Can you work these out from the model? Positions are in its coordinate system, mm. A direction names the side the tool comes from. Coordinates: 2 decimals unless noted, no trailing zeros. Order: outer loops, then holes, each group sorted by start corner. A loop starts at its lowest first (then second) coordinate and runs counter-clockwise, first axis right, second up. Notation, with made-up numbers: M -35.5,13 L -21.5,13 A10 cw -21.5,27 Z; hole C -27.5,81 d3. An arc over 180 degrees is marked long. Answer as CSV lines item,"result". Start each with the question number.
1. If we section it at A-A (x = -3.25): List the corners of the cut face in (y, z) for me, plus the area to 3 significant figures.
2. Will these pins go through, and if not, where does the flat tip stop? pin 1 (1 mm diameter, centred on x = 4.5, z = -0.5, fed in from -Y); pin 2 (0.5 mm diameter, centred on y = 1, z = -1.5, fed in from -X); pin 3 (1 mm diameter, centred on y = 3, z = 1, fed in from +X).
3. If we section it at B-B (x = 2.25): List the corners of the cut face in (y, z) for me, plus the area to 3 significant figures.
4. If we mould it in two halves opening along Z, with no side actions, what happens to faces 4 (the face through (-3.77, 1.74, 0.99)), 5 (the face through (-2.218, 2.285, 3.584)), 6 (the face through (-5, -2, 1))? For each: released by +Z, released by -Z, zero draft, split by the parting line, or undercut.
5. On a 3-axis mill with a long thin cutter (end or side, diameter ignored), from which of +Z, -Z, +X, -X, +Y, -Y can I reach the whole of each face in a straight line? I mean faces 1 (the face through (0, 0, -3)), 2 (the face through (-4, 0, 2)), 3 (the face through (8, 0, 0)). Say none if no direction works.
6. I need wall thicknesses on line 1 along Y through (x, z) = (-3.25, -1.75); line 2 along Z through (x, y) = (-2.75, -1); line 3 along X through (y, z) = (-2.25, 1.5). Which ranges of each line are inside material? Lowest first, please. Write a range as from..to.
Autodesk Inventor part; units mm, degrees
ref_plane "bolt_XY" through (0, 0, 0) normal (1, 0, 0) x (0, 0, -1)
ref_plane "bolt_YZ" through (0, 0, 0) normal (0, 0, -1) x (0, 1, 0)
ref_plane "bolt_ZX" through (0, 0, 0) normal (0, 1, 0) x (1, 0, 0)
sketch "Sketch_8" plane through (0, 0, 0) normal (0, 0, 1) x (1, 0, 0)
  line L0 (8, 0) -> (-5, 0)
  line L1 (-5, 0) -> (-5, 3.9613)
  line L2 (-5, 3.9613) -> (-4.5, 4.25)
  line L3 (-4.5, 4.25) -> (0, 4.25)
  line L4 (0, 4.25) -> (0, 2.7)
  arc A0 (0, 2.7) -> (0.2, 2.5) centre (0.2, 2.7) ccw
  line L5 (0.2, 2.5) -> (7.5095, 2.5)
  line L6 (7.5095, 2.5) -> (8, 2.0095)
  line L7 (8, 2.0095) -> (8, 0)
  line L8 (8, 0) -> (-5, 0)
revolve "Revolution1" add sketch "Sketch_8" angle 360 about axis through (8, 0, 0) along (1, 0, 0)
thread "Thread1"
sketch "Sketch2" plane through (-5, 0, 0) normal (-1, 0, 0) x (0, 0, 1)
  point P0 (0, 0)
hole "Hole1" at (-5, 0, 0) direction (1, 0, 0) diameter 4 depth 2.5 tip angle 120
sketch "Sketch_3" plane through (-5, 0, 0) normal (1, 0, 0) x (0, 0, -1)
  line L0 (-2, -1.1547) -> (0, -2.3094)
  line L1 (0, -2.3094) -> (2, -1.1547)
  line L2 (2, -1.1547) -> (2, 1.1547)
  line L3 (2, 1.1547) -> (0, 2.3094)
  line L4 (0, 2.3094) -> (-2, 1.1547)
  line L5 (-2, 1.1547) -> (-2, -1.1547)
extrude "Extrusion1" cut sketch "Sketch_3" along normal blind 2.5
ref_plane "bolt_XY" through (0, 0, 0) normal (1, 0, 0) x (0, 0, -1)
ref_plane "bolt_YZ" through (0, 0, 0) normal (0, 0, -1) x (0, 1, 0)
ref_plane "bolt_ZX" through (0, 0, 0) normal (0, 1, 0) x (1, 0, 0)
ref_plane "nut_XY" through (8, 0, 0) normal (1, 0, 0) x (0, 0, -1)
ref_plane "nut_YZ" through (8, 0, 0) normal (0, 0, -1) x (0, 1, 0)
ref_plane "nut_ZX" through (8, 0, 0) normal (0, 1, 0) x (1, 0, 0)
properties part number "CBM5-8"
Solved:
1,outline,"C 0,0 d8.5; hole M -2.31,0 L -1.15,-2 L 1.15,-2 L 2.31,0 L 1.15,2 L -1.15,2 Z"
1,area,"42.9 mm²"
2,pin 1,"y = -2.5"
2,pin 2,"x = -2.5"
2,pin 3,"x = 0"
3,outline,"C 0,0 d5"
3,area,"19.6 mm²"
4,face 4,"undercut"
4,face 5,"split by the parting line"
4,face 6,"zero draft"
5,face 1,"+X"
5,face 2,"-X"
5,face 3,"+Z, -Z, +X, +Y, -Y"
6,line 1,"-3.87..-1.3, 1.3..3.87"
6,line 2,"-4.13..-2, 2..4.13"
6,line 3,"-5..0"
